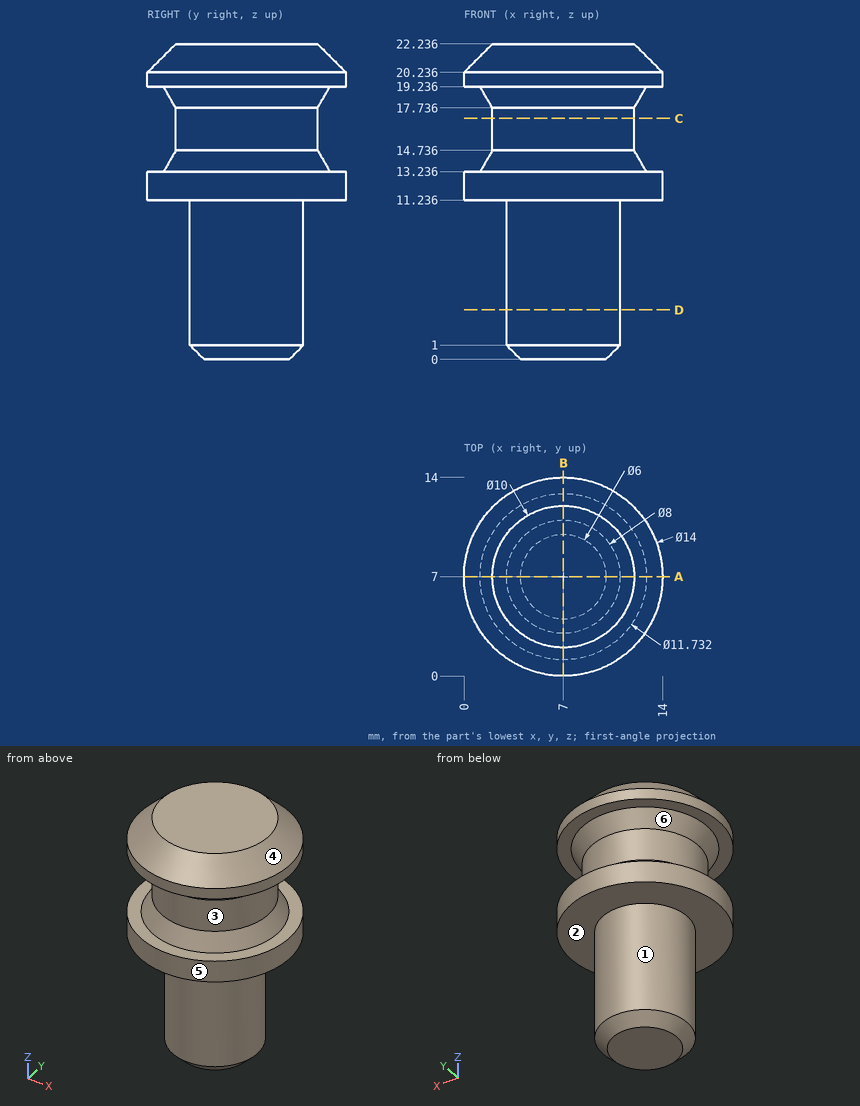
Job drawing, mm, ordinate dimensions from the low corner. One solid piece. A direction names the side the tool comes from. Give positions to 0.01 mm unless a question says otherwise; leave off trailing zeros. Write each loop counter-clockwise with the first axis right and the second up, starting at its lowest first coordinate (ties: lowest second). Pieces come first, ordered by that corner, then holes. Notation, with made-up numbers: M 25.25,66.25 L 57.25,66.25 A24 ccw 57.25,104.25 Z; hole C 79.25,66.25 d10. An arc over 180 degrees is marked long. Put each result on its own line as item: value. Start each with the question number.
(1) Mould opens along Z. For the marked faces 1, 2, 3 and 4 say: +Z half, -Z half, draft (parallel to the pull), parting line (faces both ways), or undercut.
(2) Band-saw the part on D-D, the plane z = 3.5. Write the cut outline in (x, y), and give its area (3 significant figures).
(3) Band-saw the part on A-A, the plane y = 7. Write the cut outline in (x, z), and give its area (4 significant figures).
(4) Probe L1, parallel to Y at x = 7, z = 9.25; L2, parallel to Z at x = 3, y = 3.5 (1 decimal); L3, parallel to Z at x = 5, y = 11. List the from-to ranges inside material, lowest first.
(5) Which spindle directions (+Z, -Z, +X, -X, +Y, -Y) get a long thin tool onto all of the face, cutting with end or side? Do the marked faces 5 and 6. Say none if no direction does.
(6) Flat gauge pins, fed straight in: pin 1 Ø5 at (y, z) = (9.5, 5) entering from +X; pin 2 Ø1.5 at (x, z) = (10, 15) entering from -Y; pin 3 Ø2 at (y, z) = (11.5, 8.5) entering from +X. Where does each tip first touch, or does it go through?
(7) Band-saw the part on C-C, the plane z = 17. Write the cut outline in (x, y).
Response values:
1. face 1: draft
1. face 2: -Z half
1. face 3: undercut
1. face 4: +Z half
2. outline: C 7,7 d8
2. area: 50.3 mm2
3. outline: M 0,11.24 L 3,11.24 L 3,1 L 4,0 L 10,0 L 11,1 L 11,11.24 L 14,11.24 L 14,13.24 L 12.87,13.24 L 12,14.74 L 12,17.74 L 12.87,19.24 L 14,19.24 L 14,20.24 L 12,22.24 L 2,22.24 L 0,20.24 L 0,19.24 L 1.13,19.24 L 2,17.74 L 2,14.74 L 1.13,13.24 L 0,13.24 Z
3. area: 217.5 mm2
4. L1: y = 3 to 11
4. L2: z = 11.2 to 14.2, 18.3 to 21.9
4. L3: z = 11.24 to 22.24
5. face 5: +Z, -Z
5. face 6: none
6. pin 1: stops at x = 11
6. pin 2: stops at y = 2.47
6. pin 3: stops at x = 8.94
7. outline: C 7,7 d10
